```python
from build123d import *

# Parameters (mm, degrees)
F0_W     = 50.8
F0_H     = 25.4
F1_DEPTH = 254
F2_R     = 2.5527
F3_DEPTH = 50.8
F4_R     = 2.5527
F5_DEPTH = 50.8
F6_W     = 44.45
F6_H     = 19.05
F7_DEPTH = 254


with BuildPart() as f1:
    # F0 (on Top) → F1 (new body)
    with BuildSketch(Plane.XY):
        with Locations((-0.140369, 63.959597)):
            Rectangle(F0_W, F0_H)
    extrude(amount=F1_DEPTH)

    # F2 (on face) → F3 (cut)
    with BuildSketch(Plane.XZ.offset(-51.259597)):
        with Locations((-12.840369, 241.3)):
            Circle(F2_R)
        with Locations((-12.840369, 215.9)):
            Circle(F2_R)
        with Locations((-12.840369, 190.5)):
            Circle(F2_R)
        with Locations((-12.840369, 165.1)):
            Circle(F2_R)
        with Locations((-12.840369, 139.7)):
            Circle(F2_R)
        with Locations((-12.840369, 114.3)):
            Circle(F2_R)
        with Locations((-12.840369, 88.9)):
            Circle(F2_R)
        with Locations((-12.840369, 63.5)):
            Circle(F2_R)
        with Locations((-12.840369, 38.1)):
            Circle(F2_R)
        with Locations((-12.840369, 12.7)):
            Circle(F2_R)
        with Locations((12.559631, 241.3)):
            Circle(F2_R)
        with Locations((12.559631, 215.9)):
            Circle(F2_R)
        with Locations((12.559631, 190.5)):
            Circle(F2_R)
        with Locations((12.559631, 165.1)):
            Circle(F2_R)
        with Locations((12.559631, 139.7)):
            Circle(F2_R)
        with Locations((12.559631, 114.3)):
            Circle(F2_R)
        with Locations((12.559631, 88.9)):
            Circle(F2_R)
        with Locations((12.559631, 63.5)):
            Circle(F2_R)
        with Locations((12.559631, 38.1)):
            Circle(F2_R)
        with Locations((12.559631, 12.7)):
            Circle(F2_R)
    extrude(amount=-F3_DEPTH, mode=Mode.SUBTRACT)

    # F4 (on face) → F5 (cut)
    with BuildSketch(Plane(origin=(-25.540369, 0, 0), x_dir=(0, -1, 0), z_dir=(-1, 0, 0))):
        with Locations((-63.959597, 241.3)):
            Circle(F4_R)
        with Locations((-63.959597, 215.9)):
            Circle(F4_R)
        with Locations((-63.959597, 190.5)):
            Circle(F4_R)
        with Locations((-63.959597, 165.1)):
            Circle(F4_R)
        with Locations((-63.959597, 139.7)):
            Circle(F4_R)
        with Locations((-63.959597, 114.3)):
            Circle(F4_R)
        with Locations((-63.959597, 88.9)):
            Circle(F4_R)
        with Locations((-63.959597, 63.5)):
            Circle(F4_R)
        with Locations((-63.959597, 38.1)):
            Circle(F4_R)
        with Locations((-63.959597, 12.7)):
            Circle(F4_R)
    extrude(amount=-F5_DEPTH, mode=Mode.SUBTRACT)

    # F6 (on face) → F7 (cut)
    with BuildSketch(Plane.XY.offset(254)):
        with Locations((-0.140369, 63.959597)):
            Rectangle(F6_W, F6_H)
    extrude(amount=-F7_DEPTH, mode=Mode.SUBTRACT)


solid = f1.part
```
Check sheet for the modelled part. Datum: model origin and axes. Units: mm. A direction names the side the tool comes from. Give positions to 0.01 mm unless a question says otherwise; leave off trailing zeros. Write each loop counter-clockwise with the first axis right and the second up, starting at its lowest first coordinate (ties: lowest second). Pieces come first, ordered by that corner, then holes. Notation, with made-up numbers: (73, 64) - (124, 64) arc R22 ccw to (124, 82) - close; hole circle Ø7 at (19, 42). An arc over 180 degrees is marked (long way). Answer as a JSON object with one key per item and string values. Group by question number.
1) Access from +Z, -Z, +X, -X, +Y, -Y to the whole of each face (thin tool, end or side, straight path). Record for faces 1 (the face through (-11.662, 52.825, 10.435)), 2 (the face through (0, 73.485, 129)).
2) Sectioned sample at B-B (z = 114.3). Give the number of separate pieces and of enclosed holes in the cut face, then the cut area to 3 significant figures.
3) Sectioned sample at A-A (x = -6.5). Record the cut outline in (y, z), then the cut area to 3 significant figures.
4) Sectioned sample at C-C (y = 58.5). Record the cut outline in (x, z), then the cut area to 3 significant figures.
5) Thickness scan on probe 1 along X at (y, z) = (53.4, 190.5); probe 2 along X at (y, z) = (64.25, 51); probe 3 along Y at (x, z) = (4, 215). Record the ranges inside material, lowest first. Write a range as from..to.
6) Release check for a two-part mould opening along X. For faces 3 (the face through (-13.17, 75.05, 243.83)), 4 (the face through (12.006, 75.05, 213.408)), 5 (the face through (23.65, 64.513, 35.608)), 6 (the face through (-25.54, 64, 125)) record: pulls with the +X half, pulls with the -X half, needs draft (parallel to the pull), parting line crosses it, or undercut.
7) Sectioned sample at D-D (z = 43). Record the cut outline in (x, y).
Geometry results:
{
 "1": {"face 1": "+Y, -Y", "face 2": "+Z, -Z"},
 "2": {"separate pieces": "6", "enclosed holes": "0", "area": "346 mm^2"},
 "3": {"outline": "(51.26, 0) - (54.43, 0) - (54.43, 254) - (51.26, 254) - close; (73.48, 0) - (76.66, 0) - (76.66, 254) - (73.48, 254) - close", "area": "1,610 mm^2"},
 "4": {"outline": "(-25.54, 0) - (-22.37, 0) - (-22.37, 254) - (-25.54, 254) - close; (22.08, 0) - (25.26, 0) - (25.26, 254) - (22.08, 254) - close", "area": "1,610 mm^2"},
 "5": {"probe 1": "x = -25.54..-15.39, -10.29..10.01, 15.11..25.26", "probe 2": "x = -25.54..-22.37, 22.08..25.26", "probe 3": "y = 51.26..54.43, 73.48..76.66"},
 "6": {"face 3": "undercut", "face 4": "undercut", "face 5": "needs draft", "face 6": "pulls with the -X half"},
 "7": {"outline": "(-25.54, 51.26) - (25.26, 51.26) - (25.26, 76.66) - (-25.54, 76.66) - close; hole (-22.37, 54.43) - (22.08, 54.43) - (22.08, 73.48) - (-22.37, 73.48) - close"}
}
